The listing builds one solid part. Answer for the finished solid, in the listing's coordinates (mm). A direction names the side the tool comes from. Give positions to 0.01 mm unless a question says otherwise; leave off trailing zeros. Loops run counter-clockwise (first coordinate to the right, second up) from the corner with the lowest first, then second, coordinate; pieces in that order, holes last.
Item 1: Section C-C, the plane x = 4 is taken. Give the vertices of the cut face in (y, z).
Item 2: Section B-B, the plane y = 19.5 is taken. Give the vertices of the cut face in (x, z), and give its area (3 significant figures).
Item 3: Section D-D, the plane z = 13 is taken. Give the vertices of the cut face in (x, y).
Item 4: The mould has two halves that part along Z. Classify faces 4 (the face through (37.93, 15.69, 3.62)), 5 (the face through (25.405, 27.202, 1.232)), 6 (the face through (11, 3, 25)): pulls with the +Z half, pulls with the -Z half, needs draft (parallel to the pull), parting line crosses it, or undercut.
Item 5: Each of these flat-tipped pins is pushed along its axis until it touches: pin 1 Ø3 at (x, z) = (20.5, 5) entering from +Y; pin 2 Ø3.5 at (x, z) = (-22, 2.5) entering from +Y; pin 3 Ø20 at (x, y) = (6.5, 12) entering from +Z; pin 4 Ø2.5 at (x, y) = (10.5, -4.5) entering from -Z. Where does it stop, or does it pass through?
Item 6: Section A-A, the plane y = 5 is taken. Give the vertices of the cut face in (x, z), and give its area (3 significant figures).
Item 7: A tool of negligible diameter and unlimited length cuts with its end or side. For faces 1 (the face through (43, 3.015, 4)), 2 (the face through (-18, 28.015, 15)), 3 (the face through (-3.073, 27.159, 1.232)), from which of +Z, -Z, +X, -X, +Y, -Y can it reach the whole face along a straight path? Write none if from no direction.
Item 8: Consider line 1 along Z through (x, y) = (-10, 6); line 2 along Z through (x, y) = (-20.5, 5); line 3 along X through (y, z) = (13.5, 20.5). Determine where each line is inside the solid, lowest interval first.
from build123d import *

# Parameters (mm, degrees)
BOSS_EXTRUDE1_DEPTH = 25
CUT_EXTRUDE3_START  = -25
SKETCH5_R           = 4.4
CUT_EXTRUDE3_DEPTH  = 4.8
CUT_EXTRUDE4_DEPTH  = 25
SKETCH8_W           = 50.5
SKETCH8_H           = 25.070079704
CUT_EXTRUDE5_DEPTH  = 3.5


with BuildPart() as part:
    # Sketch2 → Boss-Extrude1 (new body)
    with BuildSketch(Plane.XY):
        with BuildLine():
            Line((53.900497512, 28.014925373), (27.014667046, 28.014925373))
            ThreePointArc((27.014667046, 28.014925373), (25.389308303, 27.180347595), (25.120437848, 25.373134328))
            ThreePointArc((25.120437848, 25.373134328), (11.150497512, 5.889925373), (-2.819442823, 25.373134328))
            ThreePointArc((-2.819442823, 25.373134328), (-3.088313278, 27.180347595), (-4.713672021, 28.014925373))
            Line((-4.713672021, 28.014925373), (-31.599502488, 28.014925373))
            Line((-31.599502488, 28.014925373), (-31.599502488, -22.985074627))
            Line((-31.599502488, -22.985074627), (53.900497512, -22.985074627))
            Line((53.900497512, -22.985074627), (53.900497512, 28.014925373))
        make_face()
    extrude(amount=BOSS_EXTRUDE1_DEPTH)

    # Sketch5 → Cut-Extrude3 (cut)
    with BuildSketch(Plane.XY.offset(25).offset(CUT_EXTRUDE3_START)):
        with Locations((11.150497512, -2.910074627)):
            Circle(SKETCH5_R)
    extrude(amount=CUT_EXTRUDE3_DEPTH, mode=Mode.SUBTRACT)

    # Sketch6 → Cut-Extrude4 (cut)
    with BuildSketch(Plane(origin=(0, 28.014925373, 0), x_dir=(1, 0, 0), z_dir=(0, 1, 0))):
        Polygon((-24.599502488, 0), (-26.73851519, -7.13632431), (-14.574659319, -7.13632431), (-16.713672021, 0), align=None)
        Polygon((46.900497512, 0), (49.040087925, -7.136151124), (36.875076634, -7.136151124), (39.014667046, 0), align=None)
    extrude(amount=-CUT_EXTRUDE4_DEPTH, mode=Mode.SUBTRACT)

    # Sketch8 → Cut-Extrude5 (cut)
    with BuildSketch(Plane(origin=(0, 0, 2.5), x_dir=(-1, 0, 0), z_dir=(0, 0, -1))):
        with Locations((-11.150497512, 15.479885521)):
            Rectangle(SKETCH8_W, SKETCH8_H)
    extrude(amount=-CUT_EXTRUDE5_DEPTH, mode=Mode.SUBTRACT)


solid = part.part
Worked answers:
1. outline: (-22.99, 0) - (7.74, 0) - (7.74, 2.5) - (2.94, 2.5) - (2.94, 6) - (7.74, 6) - (7.74, 25) - (-22.99, 25) - close
2. outline: (-31.6, 0) - (-24.6, 0) - (-26.74, 7.14) - (-14.57, 7.14) - (-16.71, 0) - (-3.56, 0) - (-3.56, 2.5) - (-14.1, 2.5) - (-14.1, 6) - (-3.56, 6) - (-3.56, 25) - (-31.6, 25) - close; (25.86, 0) - (39.01, 0) - (36.88, 7.14) - (49.04, 7.14) - (46.9, 0) - (53.9, 0) - (53.9, 25) - (25.86, 25) - (25.86, 6) - (36.4, 6) - (36.4, 2.5) - (25.86, 2.5) - close
2. area: 1,190 mm2
3. outline: (-31.6, -22.99) - (53.9, -22.99) - (53.9, 28.01) - (27.01, 28.01) arc R2 ccw to (25.12, 25.37) arc R14.75 cw (long way) to (-2.82, 25.37) arc R2 ccw to (-4.71, 28.01) - (-31.6, 28.01) - close
4. face 4: undercut
4. face 5: needs draft
4. face 6: pulls with the +Z half
5. pin 1: stops at y = 10.25
5. pin 2: stops at y = 3.01
5. pin 3: stops at z = 25
5. pin 4: stops at z = 4.8
6. outline: (-31.6, 0) - (-24.6, 0) - (-26.74, 7.14) - (-14.57, 7.14) - (-16.71, 0) - (39.01, 0) - (36.88, 7.14) - (49.04, 7.14) - (46.9, 0) - (53.9, 0) - (53.9, 25) - (-31.6, 25) - close; hole (-14.1, 2.5) - (36.4, 2.5) - (36.4, 6) - (-14.1, 6) - close
6. area: 1,820 mm2
7. face 1: +Y
7. face 2: +Z, -Z, +X, -X, +Y
7. face 3: +Z, -Z
8. line 1: z = 0 to 2.5, 6 to 25
8. line 2: z = 7.14 to 25
8. line 3: x = -31.6 to -1.76, 24.06 to 53.9
